Read the model definition and answer for the solid it produces. Units are mm, in the model's axes. A direction names the side the tool comes from. Coordinates: 2 decimals unless noted, no trailing zeros. Loops run counter-clockwise (first coordinate to the right, second up) from the corner with the lowest first, then second, coordinate; pieces in that order, holes last. Notation, with made-up numbers: (8.25, 68) -> (51.25, 68) arc R23 cw to (51.25, 103) -> close; hole circle Ø5 at (-31, 73). An arc over 180 degrees is marked (long way). Answer in a Markdown table with one row per item.
```python
from build123d import *

# Parameters (mm, degrees)
SKETCH1_W            = 2.032
SKETCH1_H            = 21.59
EXTRUDE_THIN1_DEPTH  = 457.2
SKETCH2_W            = 2.286
SKETCH2_H            = 31.242
EXTRUDE_THIN2_DEPTH  = 457.2
CHAMFER1_SIZE        = 3.302
CHAMFER1_SIZE2       = 1.906410589
SKETCH3_R            = 2.3876
CUT_EXTRUDE1_DEPTH   = 2.286
LPATTERN2_COUNT      = 5
LPATTERN2_PITCH      = 203.2
LPATTERN2_COUNT_DIR2 = 5
LPATTERN2_PITCH_DIR2 = 203.2
SKETCH4_R            = 0.635
CUT_EXTRUDE2_DEPTH   = 915.93641766
LPATTERN1_COUNT      = 7
LPATTERN1_PITCH      = 3.175


with BuildPart() as part:
    # Sketch1 → Extrude-Thin1 (new, symmetric)
    with BuildSketch(Plane(origin=(0, 0, 0), x_dir=(0, 0, -1), z_dir=(1, 0, 0))):
        with Locations((-1.016, 5.461)):
            Rectangle(SKETCH1_W, SKETCH1_H)
    extrude(amount=EXTRUDE_THIN1_DEPTH, both=True)

    # Sketch2 → Extrude-Thin2 (add, symmetric)
    with BuildSketch(Plane(origin=(0, 0, 0), x_dir=(0, 0, -1), z_dir=(1, 0, 0))):
        with Locations((1.143, -15.621)):
            Rectangle(SKETCH2_W, SKETCH2_H)
    extrude(amount=EXTRUDE_THIN2_DEPTH, both=True)

    # Chamfer1
    chamfer1_edges = [part.edges().sort_by_distance(p)[0] for p in [
        (0, 16.256, 0),
    ]]
    chamfer1_side = [part.faces().sort_by_distance(p)[0] for p in [
        (0, 8.128, 0),
    ]]
    chamfer(chamfer1_edges, length=CHAMFER1_SIZE, length2=CHAMFER1_SIZE2, reference=chamfer1_side[0])

    # Sketch3 → Cut-Extrude1 (cut)
    with BuildSketch(Plane(origin=(0, 0, -2.286), x_dir=(-1, 0, 0), z_dir=(0, 0, -1))):
        with Locations((0, -15.367)):
            Circle(SKETCH3_R)
    cut_extrude1 = extrude(amount=-CUT_EXTRUDE1_DEPTH, mode=Mode.SUBTRACT)

    # LPattern2: Cut-Extrude1 5 × 5
    with Locations(*[Vector(-1, 0, 0) * (i * LPATTERN2_PITCH) + Vector(1, 0, 0) * (j * LPATTERN2_PITCH_DIR2) for i in range(LPATTERN2_COUNT) for j in range(LPATTERN2_COUNT_DIR2) if (i, j) != (0, 0)]):
        add(cut_extrude1, mode=Mode.SUBTRACT)

    # Sketch4 → Cut-Extrude2 (cut, through all)
    with BuildSketch(Plane(origin=(457.2, 0, 0), x_dir=(0, 0, -1), z_dir=(1, 0, 0))):
        with Locations((2.286, -29.972)):
            Circle(SKETCH4_R)
    cut_extrude2 = extrude(amount=-CUT_EXTRUDE2_DEPTH, mode=Mode.SUBTRACT)

    # LPattern1: Cut-Extrude2 ×7
    with Locations(*[(0, i * LPATTERN1_PITCH, 0) for i in range(1, LPATTERN1_COUNT)]):
        add(cut_extrude2, mode=Mode.SUBTRACT)


solid = part.part
```
1. Find the intervals of material crossed by probe 1 along Y at (x, z) = (0, -0.6); probe 2 along Z at (x, y) = (-222.5, -11); probe 3 along Z at (x, y) = (-92, -9), in increasing order.
A:
| item | result |
|---|---|
| probe 1 | y = -31.24 to -17.75, -12.98 to 0 |
| probe 2 | z = -1.66 to 0 |
| probe 3 | z = -2.29 to 0 |
2. A tool of negligible diameter and unlimited length cuts with its end or side. For faces 1 (the flat face through (6, -18, 0)), 2 (the flat face through (6, 5, 2.032)), from which of +Z, -Z, +X, -X, +Y, -Y can it reach the whole face along a straight path? Write none if from no direction.
A:
| item | result |
|---|---|
| face 1 | +Z, +X, -X, -Y |
| face 2 | +Z, +X, -X, +Y, -Y |
3. Given pin 1 Ø5 at (x, y) = (179.5, 5.5) entering from -Z; pin 2 Ø2 at (x, z) = (118, 1.5) entering from -Y; pin 3 Ø1 at (x, z) = (324, 0.5) entering from +Y, each flat-ended and moving along its own axis, determine where each tip first touches the part or whether it passes through.
A:
| item | result |
|---|---|
| pin 1 | stops at z = 0 |
| pin 2 | stops at y = -5.33 |
| pin 3 | stops at y = 14.69 |
4. A cutting plane is placed at A-A on x = -241. Give the vertices of the cut face in (y, z) (3 decimals).
A:
| item | result |
|---|---|
| outline | (-31.242, -2.286) -> (-30.607, -2.286) arc R0.635 cw to (-29.337, -2.286) -> (-27.432, -2.286) arc R0.635 cw to (-26.162, -2.286) -> (-24.257, -2.286) arc R0.635 cw to (-22.987, -2.286) -> (-21.082, -2.286) arc R0.635 cw to (-19.812, -2.286) -> (-17.907, -2.286) arc R0.635 cw to (-16.637, -2.286) -> (-14.732, -2.286) arc R0.635 cw to (-13.462, -2.286) -> (-11.557, -2.286) arc R0.635 cw to (-10.287, -2.286) -> (0, -2.286) -> (0, 0) -> (12.954, 0) -> (16.256, 1.906) -> (16.256, 2.032) -> (-5.334, 2.032) -> (-5.334, 0) -> (-31.242, 0) -> close |
